Work out the finished part from the listing and answer in its coordinate system (mm). Round coordinates to 2 decimals unless told otherwise and drop trailing zeros. Loops run counter-clockwise (first coordinate to the right, second up) from the corner with the lowest first, then second, coordinate; pieces in that order, holes last. Notation, with made-up numbers: (-34.5, -40) -> (18.5, -40) arc R19 cw to (18.5, -33) -> close; hole circle Ø1 at (37.25, 43). An arc over 180 degrees is marked (long way). Use CSV: the item, a comma, the result in double quotes. Start each with the question number.
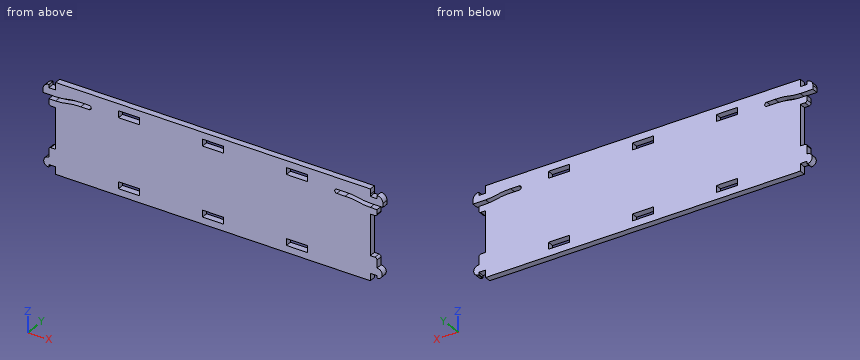
from build123d import *

# Parameters (mm, degrees)
F0_W     = 10
F0_H     = 3.25
F1_DEPTH = 3


# Not quite as in the source:
# - ends of sketch curves that miss each other by under 0.0002 mm in the source are joined


with BuildPart() as f1:
    # F0 (on Front) → F1 (new body)
    with BuildSketch(Plane.XZ):
        with BuildLine():
            Line((75, 21.5), (-75, 21.5))
            Line((-75, 21.5), (-74.9930354723, 18.0000069292))
            Line((-74.9930354723, 18.0000069292), (-78.2, 18.0000069292))
            Line((-78.2, 18.0000069292), (-78.2, 19.5000069292))
            ThreePointArc((-78.2, 19.5000069292), (-80.1867814364, 18.6729994594), (-80.999932095, 16.6805065893))
            Line((-80.999932095, 16.6805065893), (-80.9871833927, 14.85))
            Line((-80.9871833927, 14.85), (-75.0000029802, 14.85))
            add(Edge.make_bspline(
                [(-75.0000029802, 14.85), (-72.0000029802, 14.85), (-69.0064407929, 15.7236590768), (-66.0000029802, 16.1), (-63.0000029802, 16.1)],
                knots=[0, 0, 0, 0, 0.5005364838, 1, 1, 1, 1], degree=3))
            Line((-63.0000029802, 16.1), (-59.0000029802, 16.1))
            ThreePointArc((-59.0000029802, 16.1), (-58.0000029802, 15.1), (-59.0000029802, 14.1))
            Line((-59.0000029802, 14.1), (-63.0000029802, 14.1))
            add(Edge.make_bspline(
                [(-74.9999980132, 12.85), (-71.9999980132, 12.85), (-69.0064358259, 13.7236590768), (-65.9999980132, 14.1), (-63.0000029802, 14.1)],
                knots=[0, 0, 0, 0, 0.5005364838, 1, 1, 1, 1], degree=3))
            Line((-74.9999980132, 12.85), (-78.2, 12.85))
            Line((-78.2, 12.85), (-78.2, 10.75))
            ThreePointArc((-78.2, 10.75), (-77.9071067812, 10.0428932188), (-77.2, 9.75))
            Line((-77.2, 9.75), (-75, 9.75))
            Line((-75, 9.75), (-75, -9.75))
            Line((-75, -9.75), (-75, -18.0000069292))
            Line((-75, -18.0000069292), (-75, -21.5))
            Line((-75, -21.5), (75, -21.5))
            Line((75, -21.5), (75, -18.0000069292))
            Line((75, -18.0000069292), (75, -9.75))
            Line((75, -9.75), (75, 9.75))
            Line((75, 9.75), (77.2, 9.75))
            ThreePointArc((77.2, 9.75), (77.9071067812, 10.0428932188), (78.2, 10.75))
            Line((78.2, 10.75), (78.2, 12.85))
            Line((78.2, 12.85), (74.9999980132, 12.85))
            add(Edge.make_bspline(
                [(74.9999980132, 12.85), (71.9999980132, 12.85), (69.0064358259, 13.7236590768), (65.9999980132, 14.1), (62.9999980132, 14.1)],
                knots=[0, 0, 0, 0, 0.5005364838, 1, 1, 1, 1], degree=3))
            Line((62.9999980132, 14.1), (59.0000029802, 14.1))
            ThreePointArc((59.0000029802, 14.1), (58.0000029802, 15.1), (59.0000029802, 16.1))
            Line((59.0000029802, 16.1), (63.0000029802, 16.1))
            add(Edge.make_bspline(
                [(74.9710970223, 14.8500135578), (71.9903624817, 14.8528122415), (69.001599828, 15.7242650608), (66.0000029802, 16.1), (63.0000029802, 16.1)],
                knots=[0.0016101996, 0.0016101996, 0.0016101996, 0.0016101996, 0.5005364838, 1, 1, 1, 1], degree=3))
            Line((74.9710970223, 14.8500135578), (75.0000029802, 14.85))
            Line((75.0000029802, 14.85), (80.9871833927, 14.85))
            Line((80.9871833927, 14.85), (80.999932095, 16.6805065893))
            ThreePointArc((80.999932095, 16.6805065893), (80.1867814364, 18.6729994594), (78.2, 19.5000069292))
            Line((78.2, 19.5000069292), (78.2, 18.0000069292))
            Line((78.2, 18.0000069292), (74.9930354723, 18.0000069292))
            Line((74.9930354723, 18.0000069292), (75, 19))
            Line((75, 19), (75, 21.5))
        make_face()
        with Locations((-40, -16.625)):
            Rectangle(F0_W, F0_H, mode=Mode.SUBTRACT)
        with Locations((0, -16.625)):
            Rectangle(F0_W, F0_H, mode=Mode.SUBTRACT)
        with Locations((40, -16.625)):
            Rectangle(F0_W, F0_H, mode=Mode.SUBTRACT)
        with Locations((-40, 16.625)):
            Rectangle(F0_W, F0_H, mode=Mode.SUBTRACT)
        with Locations((0, 16.625)):
            Rectangle(F0_W, F0_H, mode=Mode.SUBTRACT)
        with Locations((40, 16.625)):
            Rectangle(F0_W, F0_H, mode=Mode.SUBTRACT)
        with BuildLine():
            Line((-75, -18.0000069292), (-75, -9.75))
            Line((-75, -9.75), (-77.2, -9.75))
            ThreePointArc((-77.2, -9.75), (-77.9071067812, -10.0428932188), (-78.2, -10.75))
            Line((-78.2, -10.75), (-78.2, -12.384363041))
            Line((-78.2, -12.384363041), (-78.2, -14.5073579624))
            ThreePointArc((-78.2, -14.5073579624), (-80.6617701682, -16.7497231552), (-78.4079163074, -19.2009793215))
            ThreePointArc((-78.4079163074, -19.2009793215), (-78.2614057387, -19.1453290857), (-78.2, -19.0011360528))
            Line((-78.2, -19.0011360528), (-78.2, -18.0000069292))
            Line((-78.2, -18.0000069292), (-75, -18.0000069292))
        make_face()
        with BuildLine():
            Line((77.2, -9.75), (75, -9.75))
            Line((75, -9.75), (75, -18.0000069292))
            Line((75, -18.0000069292), (78.2, -18.0000069292))
            Line((78.2, -18.0000069292), (78.2, -19.0011360528))
            ThreePointArc((78.2, -19.0011360528), (78.2614057387, -19.1453290857), (78.4079163074, -19.2009793215))
            ThreePointArc((78.4079163074, -19.2009793215), (80.6617701682, -16.7497231552), (78.2, -14.5073579624))
            Line((78.2, -14.5073579624), (78.2, -12.384363041))
            Line((78.2, -12.384363041), (78.2, -10.75))
            ThreePointArc((78.2, -10.75), (77.9071067812, -10.0428932188), (77.2, -9.75))
        make_face()
    extrude(amount=F1_DEPTH)


solid = f1.part
Q1. Each of these flat-tipped pins is pushed along its axis until it touches: pin 1 (1 mm diameter, centred on y = -1, z = 10.5, fed in from +X); pin 2 (0.8 mm diameter, centred on y = -1.5, z = 20.5, fed in from +X); pin 3 (1.5 mm diameter, centred on x = 76.5, y = -1.5, fed in from -Z). Where does it stop, or does it pass through?
Q2. Straight lines are drawn through the part: line 1 (Z direction, x = -40.5, y = -2.3); line 2 (X direction, y = -1.8, z = -17); line 3 (Z direction, x = 59.5, y = -0.65). For each, find the intervals that lie inside material, in ascending order. Write a range as from..to.
Q3. Section A-A, the plane y = -2.2 is taken. Give the number of separate pieces and of enclosed holes in the cut face, and give its area (3 significant figures).
Q4. Section B-B, the plane z = 6.5 is taken. Write down the section's boundary in (x, y).
Report:
1,pin 1,"stops at x = 78.2"
1,pin 2,"stops at x = 75"
1,pin 3,"stops at z = -18"
2,line 1,"z = -21.5..-18.25, -15..15, 18.25..21.5"
2,line 2,"x = -80.66..-45, -35..-5, 5..35, 45..80.66"
2,line 3,"z = -21.5..14.1, 16.1..21.5"
3,separate pieces,"1"
3,enclosed holes,"6"
3,area,"6,320 mm²"
4,outline,"(-75, -3) -> (75, -3) -> (75, 0) -> (-75, 0) -> close"
